```python
from build123d import *

# Parameters (mm, degrees)
F1_DEPTH = 5


with BuildPart() as f1:
    # F0 (on Front) → F1 (new body)
    with BuildSketch(Plane.XZ):
        with BuildLine():
            Line((-1.498945, 9.94375), (-1.498945, 19.94375))
            ThreePointArc((-1.498945, 19.94375), (-7.653669, 18.477591), (-13.042447, 15.162275))
            Line((-13.042447, 15.162275), (-5.971379, 8.091207))
            Line((-5.971379, 8.091207), (-8.091207, 5.971379))
            Line((-8.091207, 5.971379), (-15.162275, 13.042447))
            ThreePointArc((-15.162275, 13.042447), (-18.477591, 7.653669), (-19.94375, 1.498945))
            Line((-19.94375, 1.498945), (-9.94375, 1.498945))
            Line((-9.94375, 1.498945), (-9.94375, -1.498945))
            Line((-9.94375, -1.498945), (-19.94375, -1.498945))
            ThreePointArc((-19.94375, -1.498945), (-18.477591, -7.653669), (-15.162275, -13.042447))
            Line((-15.162275, -13.042447), (-8.091207, -5.971379))
            Line((-8.091207, -5.971379), (-5.971379, -8.091207))
            Line((-5.971379, -8.091207), (-13.042447, -15.162275))
            ThreePointArc((-13.042447, -15.162275), (-7.653669, -18.477591), (-1.498945, -19.94375))
            Line((-1.498945, -19.94375), (-1.498945, -9.94375))
            Line((-1.498945, -9.94375), (1.498945, -9.94375))
            Line((1.498945, -9.94375), (1.498945, -19.94375))
            ThreePointArc((1.498945, -19.94375), (7.653669, -18.477591), (13.042447, -15.162275))
            Line((13.042447, -15.162275), (5.971379, -8.091207))
            Line((5.971379, -8.091207), (8.091207, -5.971379))
            Line((8.091207, -5.971379), (15.162275, -13.042447))
            ThreePointArc((15.162275, -13.042447), (18.477591, -7.653669), (19.94375, -1.498945))
            Line((19.94375, -1.498945), (9.94375, -1.498945))
            Line((9.94375, -1.498945), (9.94375, 1.498945))
            Line((9.94375, 1.498945), (19.94375, 1.498945))
            ThreePointArc((19.94375, 1.498945), (18.477591, 7.653669), (15.162275, 13.042447))
            Line((15.162275, 13.042447), (8.091207, 5.971379))
            Line((8.091207, 5.971379), (5.971379, 8.091207))
            Line((5.971379, 8.091207), (13.042447, 15.162275))
            ThreePointArc((13.042447, 15.162275), (7.653669, 18.477591), (1.498945, 19.94375))
            Line((1.498945, 19.94375), (1.498945, 9.94375))
            Line((1.498945, 9.94375), (-1.498945, 9.94375))
        make_face()
    extrude(amount=F1_DEPTH)


solid = f1.part
```
Build history of the part. All positions in model axes, mm. A direction names the side the tool comes from. Give positions to 0.01 mm unless a question says otherwise; leave off trailing zeros. Order: outer loops, then holes, each group sorted by start corner. A loop starts at its lowest first (then second) coordinate and runs counter-clockwise, first axis right, second up. Notation, with made-up numbers: M -16,78.25 L -7,78.25 A33 cw -7,110.25 Z; hole C 35,45.25 d3. An arc over 180 degrees is marked long. Write item = value, one per line. Start each with the question number.
(1) Pin check, flat tips, straight feed: pin 1 Ø1.5 at (x, y) = (14, -3.5) entering from -Z; pin 2 Ø1.5 at (y, z) = (-3, -14) entering from -X; pin 3 Ø1.5 at (x, z) = (-12.5, 14) entering from +Y; pin 4 Ø1.5 at (y, z) = (-2, 16) entering from -X. Stop position of each tip, or through.
(2) Slice it at C-C on z = 7.5. Write the cut outline in (x, y), plus the area to 3 significant figures.
(3) Two-plate mould, pull along Z, no slides. Class faces 6 (the cylindrical face through (7.74, -2.46, 18.44)), 7 (the cylindrical face through (7.6, -2.5, -18.5)), 8 (the flat face through (-11.68, -2.46, -9.56)): released by +Z, released by -Z, zero draft, split by the parting line, or undercut.
(4) Probe L1, parallel to Z at x = -7, y = -3.8 (3 decimals); L2, parallel to Z at x = 6.5, y = -2.8; L3, parallel to X at y = -1.85, z = -9. List the from-to ranges inside material, lowest first. Write a range as [from, to].
(5) Slice it at D-D on z = -12. Write the cut outline in (x, y).
(6) Which spindle directions (+Z, -Z, +X, -X, +Y, -Y) get a long thin tool onto all of the face, cutting with end or side? Do faces 1 (the flat face through (15, -2, -1.499)), 2 (the flat face through (1.499, -2, 15)), 3 (the flat face through (1.499, -2, -15)), 4 (the flat face through (-11.58, -2.46, 9.46)), 5 (the flat face through (-15, -2, 1.499)). Say none if no direction does.
(7) Slice it at A-A on z = -16. Write the cut outline in (x, y), plus the area to 3 significant figures.
Responses:
q1.pin_1 = -12.63
q1.pin_2 = -12.63
q1.pin_3 = 0
q1.pin_4 = -12.94
q2.outline = M -18.54,-5 L -9.62,-5 L -9.62,0 L -18.54,0 Z; M -6.56,-5 L 6.56,-5 L 6.56,0 L -6.56,0 Z; M 9.62,-5 L 18.54,-5 L 18.54,0 L 9.62,0 Z
q2.area = 155 mm2
q3.face_6 = released by +Z
q3.face_7 = released by -Z
q3.face_8 = undercut
q4.L1 = [-18.735, -9.12], [-7.063, 7.063], [9.12, 18.735]
q4.L2 = [-18.91, -8.62], [-7.56, 7.56], [8.62, 18.91]
q4.L3 = [-17.86, -11.12], [-6.88, 6.88], [11.12, 17.86]
q5.outline = M -16,-5 L -14.12,-5 L -14.12,0 L -16,0 Z; M -9.88,-5 L -1.5,-5 L -1.5,0 L -9.88,0 Z; M 1.5,-5 L 9.88,-5 L 9.88,0 L 1.5,0 Z; M 14.12,-5 L 16,-5 L 16,0 L 14.12,0 Z
q6.face_1 = +X, +Y, -Y
q6.face_2 = +Z, +Y, -Y
q6.face_3 = -Z, +Y, -Y
q6.face_4 = +Y, -Y
q6.face_5 = -X, +Y, -Y
q7.outline = M -12,-5 L -1.5,-5 L -1.5,0 L -12,0 Z; M 1.5,-5 L 12,-5 L 12,0 L 1.5,0 Z
q7.area = 105 mm2
